CAD build for the part. Positions are in the model's coordinates, mm. Face numbers are marked on the shaded views. A direction names the side the tool comes from. Give positions to 0.01 mm unless a question says otherwise; leave off trailing zeros. Write each loop counter-clockwise with the first axis right and the second up, starting at its lowest first coordinate (ties: lowest second). Pieces come first, ordered by that corner, then holes. Notation, with made-up numbers: M 33,64 L 79,64 A27 ccw 79,92 Z; hole C -26,-17.5 d11. An arc over 180 degrees is marked long. One line per question, with ' | ' between items. Start each with the question number.
1. Flat gauge pins, fed straight in: pin 1 (3 mm diameter, centred on x = 8, z = 0, fed in from -Y); pin 2 (1 mm diameter, centred on x = -10.5, z = 4.5, fed in from +Y); pin 3 (3 mm diameter, centred on y = 4, z = 8, fed in from +X). Where does each tip first touch, or does it go through?
2. Cut at B-B, the plane z = 0.5. Write the cut outline in (x, y).
3. Which spindle directions (+Z, -Z, +X, -X, +Y, -Y) get a long thin tool onto all of the face, cutting with end or side? Do the marked faces 1, 2 and 3. Say none if no direction does.
4. Wall check: L1, parallel to Z at x = -8, y = 4.75; L2, parallel to Y at x = 8.5, z = -1.75; L3, parallel to Y at x = -5.5, z = 13.75. Give the ranges that are in metal, low to high.
5. Pull direction X, two halves, no side cores. Call the marked faces 4, 5 and 6: released by +X, released by -X, zero draft, split by the parting line, or undercut.
6. Cut at A-A, the plane x = 0. Write the cut outline in (y, z), then the cut area to 4 significant figures.
7. Cut at C-C, the plane y = 7.5. Write the cut outline in (x, z), then the cut area to 3 significant figures.
8. Cut at D-D, the plane z = 8. Write the cut outline in (x, y).
```python
from build123d import *

# Parameters (mm, degrees)
SKETCH1_R           = 15
BOSS_EXTRUDE1_DEPTH = 10
SKETCH2_R           = 1.95
BOSS_EXTRUDE2_DEPTH = 2
CUT_EXTRUDE1_DEPTH  = 2
SKETCH4_R           = 1.35
CUT_EXTRUDE2_DEPTH  = 24.452078799
CIRPATTERN2_COUNT   = 4
CIRPATTERN3_COUNT   = 4
SKETCH5_R           = 3
CUT_EXTRUDE3_DEPTH  = 5
SKETCH6_R           = 1.35
CUT_EXTRUDE4_DEPTH  = 23.338307904


with BuildPart() as part:
    # Sketch1 → Boss-Extrude1 (new body)
    with BuildSketch(Plane(origin=(0, 0, 0), x_dir=(1, 0, 0), z_dir=(0, 1, 0))):
        with Locations(Location((0, 0, 0), (0, 0, 270))):
            Circle(SKETCH1_R)
    extrude(amount=BOSS_EXTRUDE1_DEPTH)

    # Sketch2 → Boss-Extrude2 (add)
    with BuildSketch(Plane(origin=(0, 10, 0), x_dir=(1, 0, 0), z_dir=(0, 1, 0))):
        with Locations(Location((4.179388408, 4.179388408, 0), (0, 0, 270))):
            Circle(SKETCH2_R)
    boss_extrude2 = extrude(amount=BOSS_EXTRUDE2_DEPTH)

    # Sketch3 → Cut-Extrude1 (cut)
    with BuildSketch(Plane.XZ):
        Polygon((-2.05, 10.5), (2.05, 10.5), (2.05, 2), (10.55, 2), (10.55, -2.1), (2.05, -2.1), (2.05, -10.6), (-2.05, -10.6), (-2.05, -2.1), (-10.55, -2.1), (-10.55, 2), (-2.05, 2), align=None)
    extrude(amount=-CUT_EXTRUDE1_DEPTH, mode=Mode.SUBTRACT)

    # Sketch4 → Cut-Extrude2 (cut, through all)
    with BuildSketch(Plane.XZ.offset(-2)):
        with Locations(Location((0, 8, 0), (0, 0, 270))):
            Circle(SKETCH4_R)
    cut_extrude2 = extrude(amount=-CUT_EXTRUDE2_DEPTH, mode=Mode.SUBTRACT)

    # CirPattern2: Cut-Extrude2 ×4 about axis
    cirpattern2_axis = Axis((0, 0, 0), (0, 1, 0))
    for i in range(1, CIRPATTERN2_COUNT):
        add(cut_extrude2.rotate(cirpattern2_axis, i * 360 / CIRPATTERN2_COUNT), mode=Mode.SUBTRACT)

    # CirPattern3: Boss-Extrude2 ×4 about axis
    cirpattern3_axis = Axis((0, 0, 0), (0, 1, 0))
    for i in range(1, CIRPATTERN3_COUNT):
        add(boss_extrude2.rotate(cirpattern3_axis, i * 360 / CIRPATTERN3_COUNT))

    # Sketch5 → Cut-Extrude3 (cut)
    with BuildSketch(Plane.XZ.offset(-2)):
        with Locations(Location((0, 0, 0), (0, 0, 270))):
            Circle(SKETCH5_R)
    extrude(amount=-CUT_EXTRUDE3_DEPTH, mode=Mode.SUBTRACT)

    # Sketch6 → Cut-Extrude4 (cut, through all)
    with BuildSketch(Plane.XZ.offset(-7)):
        with Locations(Location((0, 0, 0), (0, 0, 270))):
            Circle(SKETCH6_R)
    extrude(amount=-CUT_EXTRUDE4_DEPTH, mode=Mode.SUBTRACT)


solid = part.part
```
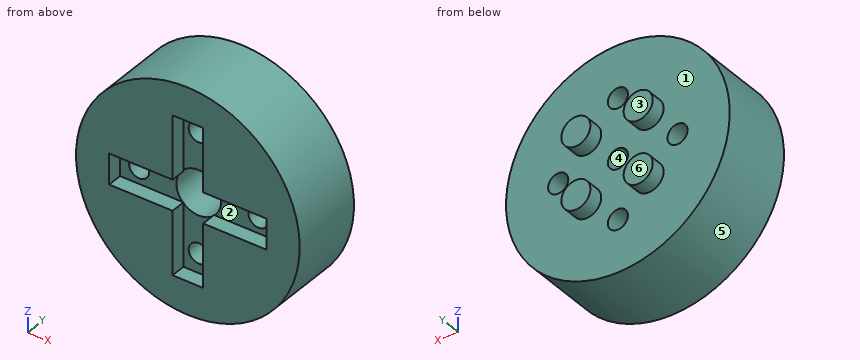
Here are the results:
1) pin 1: y = 2 | pin 2: y = 10 | pin 3: x = 13.52
2) outline: M -14.99,0 L -10.55,0 L -10.55,2 L -9.25,2 L -9.25,10 L -14.99,10 Z; M -6.75,2 L -2.96,2 L -2.96,7 L -1.25,7 L -1.25,10 L -6.75,10 Z; M 1.25,7 L 2.96,7 L 2.96,2 L 6.75,2 L 6.75,10 L 1.25,10 Z; M 9.25,2 L 10.55,2 L 10.55,0 L 14.99,0 L 14.99,10 L 9.25,10 Z
3) face 1: +Y | face 2: -Y | face 3: +Z, -Z, +X, -X, +Y
4) L1: -12.69 to -1.35, 1.35 to 12.69 | L2: 2 to 10 | L3: 0 to 10
5) face 4: undercut | face 5: split by the parting line | face 6: zero draft
6) outline: M 0,-15 L 10,-15 L 10,-9.35 L 2,-9.35 L 2,-10.6 L 0,-10.6 Z; M 0,10.5 L 2,10.5 L 2,9.35 L 10,9.35 L 10,15 L 0,15 Z; M 2,-6.65 L 10,-6.65 L 10,-1.35 L 7,-1.35 L 7,-3 L 2,-3 Z; M 2,3 L 7,3 L 7,1.35 L 10,1.35 L 10,6.65 L 2,6.65 Z | area: 176.5 mm^2
7) outline: C 0,0 d30; hole C -8,0 d2.7; hole C 0,-8 d2.7; hole C 0,0 d2.7; hole C 0,8 d2.7; hole C 8,0 d2.7 | area: 678 mm^2
8) outline: M -12.69,0 L -2.05,0 L -2.05,2 L -1.35,2 L -1.35,10 L -12.69,10 Z; M 1.35,2 L 2.05,2 L 2.05,0 L 12.69,0 L 12.69,10 L 1.35,10 Z
